from build123d import *

# Parameters (mm, degrees)
SKETCH_1_R          = 10
EXTRUDE_1_DEPTH     = 20
SKETCH_2_R          = 45
EXTRUDE_2_DEPTH     = 20
CUT_EXTRUDE_1_DEPTH = 20


with BuildPart() as part:
    # 草图1 → 凸台-拉伸1 (new body)
    with BuildSketch(Plane(origin=(0, 0, 0), x_dir=(0, 0, -1), z_dir=(1, 0, 0))):
        Circle(SKETCH_1_R)
    extrude(amount=EXTRUDE_1_DEPTH)

    # 草图2 → 凸台-拉伸2 (add)
    with BuildSketch(Plane(origin=(20, 0, 0), x_dir=(0, 0, -1), z_dir=(1, 0, 0))):
        Circle(SKETCH_2_R)
    extrude(amount=EXTRUDE_2_DEPTH)

    # 草图3 → 切除-拉伸1 (cut)
    with BuildSketch(Plane.ZY.offset(-20)):
        with BuildLine():
            Line((-9.705714191, 36.222218486), (-3.882285677, 14.488887394))
            ThreePointArc((-3.882285677, 14.488887394), (0, 15), (3.882285677, 14.488887394))
            Line((3.882285677, 14.488887394), (9.705714191, 36.222218486))
            ThreePointArc((9.705714191, 36.222218486), (0, 37.5), (-9.705714191, 36.222218486))
        make_face()
        with BuildLine():
            Line((26.516504294, 26.516504294), (10.606601718, 10.606601718))
            ThreePointArc((10.606601718, 10.606601718), (12.990381057, 7.5), (14.488887394, 3.882285677))
            Line((14.488887394, 3.882285677), (36.222218486, 9.705714191))
            ThreePointArc((36.222218486, 9.705714191), (32.475952642, 18.75), (26.516504294, 26.516504294))
        make_face()
        with BuildLine():
            Line((36.222218486, -9.705714191), (14.488887394, -3.882285677))
            ThreePointArc((14.488887394, -3.882285677), (12.990381057, -7.5), (10.606601718, -10.606601718))
            Line((10.606601718, -10.606601718), (26.516504294, -26.516504294))
            ThreePointArc((26.516504294, -26.516504294), (32.475952642, -18.75), (36.222218486, -9.705714191))
        make_face()
        with BuildLine():
            Line((9.705714191, -36.222218486), (3.882285677, -14.488887394))
            ThreePointArc((3.882285677, -14.488887394), (0, -15), (-3.882285677, -14.488887394))
            Line((-3.882285677, -14.488887394), (-9.705714191, -36.222218486))
            ThreePointArc((-9.705714191, -36.222218486), (0, -37.5), (9.705714191, -36.222218486))
        make_face()
        with BuildLine():
            Line((-26.516504294, -26.516504294), (-10.606601718, -10.606601718))
            ThreePointArc((-10.606601718, -10.606601718), (-12.990381057, -7.5), (-14.488887394, -3.882285677))
            Line((-14.488887394, -3.882285677), (-36.222218486, -9.705714191))
            ThreePointArc((-36.222218486, -9.705714191), (-32.475952642, -18.75), (-26.516504294, -26.516504294))
        make_face()
        with BuildLine():
            Line((-36.222218486, 9.705714191), (-14.488887394, 3.882285677))
            ThreePointArc((-14.488887394, 3.882285677), (-12.990381057, 7.5), (-10.606601718, 10.606601718))
            Line((-10.606601718, 10.606601718), (-26.516504294, 26.516504294))
            ThreePointArc((-26.516504294, 26.516504294), (-32.475952642, 18.75), (-36.222218486, 9.705714191))
        make_face()
    extrude(amount=-CUT_EXTRUDE_1_DEPTH, mode=Mode.SUBTRACT)


solid = part.part
CAD build for the part. Positions are in the model's coordinates, mm. A direction names the side the tool comes from. Give positions to 0.01 mm unless a question says otherwise; leave off trailing zeros. Order: outer loops, then holes, each group sorted by start corner. A loop starts at its lowest first (then second) coordinate and runs counter-clockwise, first axis right, second up. Notation, with made-up numbers: (62, 23) -> (89, 23) arc R27 ccw to (89, 55) -> close; hole circle Ø2 at (71.5, 29). An arc over 180 degrees is marked (long way). Return JSON: item names as keys, results as strings.
Q1. Which spindle directions (+Z, -Z, +X, -X, +Y, -Y) get a long thin tool onto all of the face, cutting with end or side? Do faces 1 (the face through (40, 1, 1)), 2 (the face through (29.86, 18.631, 32.544)). Say none if no direction does.
Working result:
{"face 1": "+Z, -Z, +X, +Y, -Y", "face 2": "+X, -X"}
Q2. Drill centre lines: line 1 (Y direction, x = 22, z = 22); line 2 (Y direction, x = 36.5, z = 24); line 3 (X direction, y = -14, z = 7.5). Where is each one in solid material? Low to high.
Working result:
{"line 1": "-39.26 to -22, -5.89 to 5.89, 22 to 39.26", "line 2": "-38.07 to -24, -6.43 to 6.43, 24 to 38.07", "line 3": "20 to 40"}
Q3. Mould opens along Y. For faces 3 (the face through (9.86, -9.76, 2.17)), 4 (the face through (20, -9, -9)), 5 (the face through (29.86, -25.203, -6.753)) say: pulls with the +Y half, pulls with the -Y half, needs draft (parallel to the pull), parting line crosses it, or undercut.
Working result:
{"face 3": "parting line crosses it", "face 4": "needs draft", "face 5": "undercut"}
Q4. Saw through at C-C (y = -7). Write the cut outline in (x, z), then the cut area to 3 significant figures.
Working result:
{"outline": "(0, -7.14) -> (20, -7.14) -> (20, -13.27) -> (40, -13.27) -> (40, 13.27) -> (20, 13.27) -> (20, 7.14) -> (0, 7.14) -> close; (20, -44.45) -> (40, -44.45) -> (40, -26.12) -> (20, -26.12) -> close; (20, 26.12) -> (40, 26.12) -> (40, 44.45) -> (20, 44.45) -> close", "area": "1,550 mm²"}
Q5. Saw through at A-A (z = 0). Write the cut outline in (x, y), then the cut area to 3 significant figures.
Working result:
{"outline": "(0, -10) -> (20, -10) -> (20, -15) -> (40, -15) -> (40, 15) -> (20, 15) -> (20, 10) -> (0, 10) -> close; (20, -45) -> (40, -45) -> (40, -37.5) -> (20, -37.5) -> close; (20, 37.5) -> (40, 37.5) -> (40, 45) -> (20, 45) -> close", "area": "1,300 mm²"}
Q6. Flat gauge pins, fed straight in: pin 1 (1.5 mm diameter, centred on x = 32, y = 6, fed in from -Z); pin 2 (8 mm diameter, centred on y = 20.5, z = 7.5, fed in from -X); pin 3 (3 mm diameter, centred on x = 21, z = 17, fed in from -Y). Where does each tip first touch, or does it go through?
Working result:
{"pin 1": "z = -44.69", "pin 2": "x = 20", "pin 3": "y = -42.25"}
Q7. Saw through at B-B (x = 34.5). Write the cut outline in (y, z).
Working result:
{"outline": "circle Ø90 at (0, 0); hole (-36.22, -9.71) -> (-14.49, -3.88) arc R15 cw to (-14.49, 3.88) -> (-36.22, 9.71) arc R37.5 ccw to start; hole (-26.52, -26.52) arc R37.5 ccw to (-9.71, -36.22) -> (-3.88, -14.49) arc R15 cw to (-10.61, -10.61) -> close; hole (-26.52, 26.52) -> (-10.61, 10.61) arc R15 cw to (-3.88, 14.49) -> (-9.71, 36.22) arc R37.5 ccw to start; hole (3.88, -14.49) -> (9.71, -36.22) arc R37.5 ccw to (26.52, -26.52) -> (10.61, -10.61) arc R15 cw to start; hole (3.88, 14.49) arc R15 cw to (10.61, 10.61) -> (26.52, 26.52) arc R37.5 ccw to (9.71, 36.22) -> close; hole (14.49, -3.88) -> (36.22, -9.71) arc R37.5 ccw to (36.22, 9.71) -> (14.49, 3.88) arc R15 cw to start"}
Q8. Saw through at D-D (y = 32). Write the cut outline in (x, z), then the cut area to 3 significant figures.
Working result:
{"outline": "(20, -31.64) -> (40, -31.64) -> (40, -8.57) -> (20, -8.57) -> close; (20, 8.57) -> (40, 8.57) -> (40, 31.64) -> (20, 31.64) -> close", "area": "923 mm²"}
